Work out the finished part from the listing and answer in its coordinate system (mm). A direction names the side the tool comes from. Round coordinates to 2 decimals unless told otherwise and drop trailing zeros. Order: outer loops, then holes, each group sorted by start corner. A loop starts at its lowest first (then second) coordinate and runs counter-clockwise, first axis right, second up. Notation, with made-up numbers: (88.25, 88.25) - (133.25, 88.25) arc R13 ccw to (133.25, 105.25) - close; hole circle Ø8 at (54, 16). An arc over 180 degrees is marked (long way). Answer in a Markdown table with one row per item.
from build123d import *

# Parameters (mm, degrees)
SKETCH1_W           = 33
SKETCH1_H           = 33
SKETCH1_R           = 1.5
BOSS_EXTRUDE1_DEPTH = 0.5
SKETCH2_W           = 21
SKETCH2_H           = 7
SKETCH2_W_2         = 10.5
SKETCH2_W_3         = 9.939031212
SKETCH2_H_2         = 3.481183521
BOSS_EXTRUDE2_DEPTH = 10
SKETCH3_W           = 5.42424951
SKETCH3_H           = 5.162839894
SKETCH3_W_2         = 7.058059603
SKETCH3_H_2         = 2.81015336
SKETCH3_W_3         = 3.790439417
SKETCH3_H_3         = 3.365648792
BOSS_EXTRUDE3_DEPTH = 2
SKETCH4_W           = 3.136915379
SKETCH4_H           = 2.744800957
BOSS_EXTRUDE4_DEPTH = 7
CUT_EXTRUDE1_DEPTH  = 24


with BuildPart() as part:
    # Sketch1 → Boss-Extrude1 (new, symmetric)
    with BuildSketch(Plane(origin=(0, 0, 0), x_dir=(1, 0, 0), z_dir=(0, 1, 0))):
        Rectangle(SKETCH1_W, SKETCH1_H)
        with Locations(Location((-13.5, 13.5, 0), (0, 0, 270))):
            Circle(SKETCH1_R, mode=Mode.SUBTRACT)
        with Locations(Location((-13.5, -13.5, 0), (0, 0, 90))):
            Circle(SKETCH1_R, mode=Mode.SUBTRACT)
        with Locations(Location((13.5, -13.5, 0), (0, 0, 270))):
            Circle(SKETCH1_R, mode=Mode.SUBTRACT)
        with Locations(Location((13.5, 13.5, 0), (0, 0, 90))):
            Circle(SKETCH1_R, mode=Mode.SUBTRACT)
    extrude(amount=BOSS_EXTRUDE1_DEPTH, both=True)

    # Sketch2 → Boss-Extrude2 (add)
    with BuildSketch(Plane(origin=(0, 0.5, 0), x_dir=(1, 0, 0), z_dir=(0, 1, 0))):
        with Locations((0, 12.5)):
            Rectangle(SKETCH2_W, SKETCH2_H)
        with Locations((-5.25, -12.5)):
            Rectangle(SKETCH2_W_2, SKETCH2_H)
        with Locations((-9.842504173, -6.265483719)):
            Rectangle(SKETCH2_W_3, SKETCH2_H_2)
    extrude(amount=BOSS_EXTRUDE2_DEPTH)

    # Sketch3 → Boss-Extrude3 (add)
    with BuildSketch(Plane(origin=(0, 0.5, 0), x_dir=(1, 0, 0), z_dir=(0, 1, 0))):
        with Locations((3.888468022, -8.953279311)):
            Rectangle(SKETCH3_W, SKETCH3_H)
        with Locations((5.685659125, 6.012421143)):
            Rectangle(SKETCH3_W_2, SKETCH3_H_2)
        with Locations((-7.842288448, -1.682824396)):
            Rectangle(SKETCH3_W_3, SKETCH3_H_3)
    extrude(amount=BOSS_EXTRUDE3_DEPTH)

    # Sketch4 → Boss-Extrude4 (add)
    with BuildSketch(Plane(origin=(0, 0.5, 0), x_dir=(1, 0, 0), z_dir=(0, 1, 0))):
        with Locations((13.397242764, 5.914392538)):
            Rectangle(SKETCH4_W, SKETCH4_H)
    extrude(amount=BOSS_EXTRUDE4_DEPTH)

    # Sketch5 → Cut-Extrude1 (cut)
    with BuildSketch(Plane(origin=(10.5, 0, 0), x_dir=(0, 0, -1), z_dir=(1, 0, 0))):
        Polygon((-16, 10.5), (-16, 7.5), (-14.7, 10.5), align=None)
        Polygon((-10.3, 10.5), (-9, 10.5), (-9, 7.5), align=None)
        Polygon((9, 7.5), (10.3, 10.5), (9, 10.5), align=None)
        Polygon((16, 10.5), (14.7, 10.5), (16, 7.5), align=None)
    extrude(amount=-CUT_EXTRUDE1_DEPTH, mode=Mode.SUBTRACT)


solid = part.part
1) The mould has two halves that part along Z. Classify faces 6 (the face through (4, 1, 11.535)), 7 (the face through (10.5, 5, -12)), 8 (the face through (-5.18, 8.98, 9.64)), 9 (the face through (-10, 5, 8.006)): released by +Z, released by -Z, zero draft, split by the parting line, or undercut.
Filled in:
| item | result |
|---|---|
| face 6 | released by +Z |
| face 7 | zero draft |
| face 8 | undercut |
| face 9 | undercut |
2) Find section D-D, the plane y = 3.75. Give the vertices of the cut face in (x, z).
Filled in:
| item | result |
|---|---|
| outline | (-14.81, 4.52) - (-4.87, 4.52) - (-4.87, 8.01) - (-14.81, 8.01) - close; (-10.5, -16) - (10.5, -16) - (10.5, -9) - (-10.5, -9) - close; (-10.5, 9) - (0, 9) - (0, 16) - (-10.5, 16) - close; (11.83, -7.29) - (14.97, -7.29) - (14.97, -4.54) - (11.83, -4.54) - close |
3) Find section C-C, the plane z = -13.5. Give the vertices of the cut face in (x, y), then the cut area to 3 significant figures.
Filled in:
| item | result |
|---|---|
| outline | (-16.5, -0.5) - (-15, -0.5) - (-15, 0.5) - (-16.5, 0.5) - close; (-12, -0.5) - (12, -0.5) - (12, 0.5) - (10.5, 0.5) - (10.5, 10.5) - (-10.5, 10.5) - (-10.5, 0.5) - (-12, 0.5) - close; (15, -0.5) - (16.5, -0.5) - (16.5, 0.5) - (15, 0.5) - close |
| area | 237 mm^2 |
4) Find section B-B, the plane x = 13.5. Give the vertices of the cut face in (y, z), then the cut area to 3 significant figures.
Filled in:
| item | result |
|---|---|
| outline | (-0.5, -16.5) - (0.5, -16.5) - (0.5, -15) - (-0.5, -15) - close; (-0.5, -12) - (0.5, -12) - (0.5, -7.29) - (7.5, -7.29) - (7.5, -4.54) - (0.5, -4.54) - (0.5, 12) - (-0.5, 12) - close; (-0.5, 15) - (0.5, 15) - (0.5, 16.5) - (-0.5, 16.5) - close |
| area | 46.2 mm^2 |
5) Which of the six approach directions +Z, -Z, +X, -X, +Y, -Y give full straight-line access (tool end or side, diameter ignored) to faces 1 (the face through (-10.5, 5, 13)), 2 (the face through (0, 4, -9)), 3 (the face through (-5, 4, 9)), 4 (the face through (-5.947, 1, 2)), 5 (the face through (0, 4, -16))?
Filled in:
| item | result |
|---|---|
| face 1 | +Z, -X, +Y |
| face 2 | +X, -X, +Y |
| face 3 | -X, +Y |
| face 4 | +X, +Y |
| face 5 | -Z, +X, -X, +Y |
6) Find the intervals of material crossed by probe 1 along Z at (x, y) = (-6, 7); probe 2 along X at (y, z) = (0.15, -13.5); probe 3 along Z at (x, y) = (-9, 9), in increasing order. Write a range as from..to.
Filled in:
| item | result |
|---|---|
| probe 1 | z = -16..-9, 4.52..8.01, 9..16 |
| probe 2 | x = -16.5..-15, -12..12, 15..16.5 |
| probe 3 | z = -15.35..-9.65, 4.52..8.01, 9.65..15.35 |
7) Each of these flat-tipped pins is pushed along its axis until it touches: pin 1 (4 mm diameter, centred on y = 4, z = 0.5, fed in from -X); pin 2 (2 mm diameter, centred on x = 5.5, y = 2, fed in from -Z); pin 3 (2 mm diameter, centred on x = 5.5, z = -6.5, fed in from +Y). Where does it stop, or does it pass through?
Filled in:
| item | result |
|---|---|
| pin 1 | stops at x = -9.74 |
| pin 2 | stops at z = -16 |
| pin 3 | stops at y = 2.5 |
8) Find section A-A, the plane y = 1.5. Give the vertices of the cut face in (x, z), then the cut area to 3 significant figures.
Filled in:
| item | result |
|---|---|
| outline | (-14.81, 4.52) - (-4.87, 4.52) - (-4.87, 8.01) - (-14.81, 8.01) - close; (-10.5, -16) - (10.5, -16) - (10.5, -9) - (-10.5, -9) - close; (-10.5, 9) - (0, 9) - (0, 16) - (-10.5, 16) - close; (-9.74, 0) - (-5.95, 0) - (-5.95, 3.37) - (-9.74, 3.37) - close; (1.18, 6.37) - (6.6, 6.37) - (6.6, 11.53) - (1.18, 11.53) - close; (2.16, -7.42) - (9.21, -7.42) - (9.21, -4.61) - (2.16, -4.61) - close; (11.83, -7.29) - (14.97, -7.29) - (14.97, -4.54) - (11.83, -4.54) - close |
| area | 324 mm^2 |
